from build123d import *

# Parameters (mm, degrees)
SKETCH_1_R          = 2.5
EXTRUDE_1_DEPTH     = 3
SKETCH_2_R          = 1.5
EXTRUDE_2_DEPTH     = 6
CUT_EXTRUDE_1_DEPTH = 2
CHAMFER_1_SIZE      = 0.3
FILLET_1_R          = 0.3


with BuildPart() as part:
    # 草图1 → 凸台-拉伸1 (new body)
    with BuildSketch(Plane.XY):
        Circle(SKETCH_1_R)
    extrude(amount=EXTRUDE_1_DEPTH)

    # 草图2 → 凸台-拉伸2 (add)
    with BuildSketch(Plane(origin=(0, 0, 0), x_dir=(-1, 0, 0), z_dir=(0, 0, -1))):
        Circle(SKETCH_2_R)
    extrude(amount=EXTRUDE_2_DEPTH)

    # 草图3 → 切除-拉伸1 (cut)
    with BuildSketch(Plane.XY.offset(3)):
        Polygon((1.443375673, 0), (0.721687836, 1.25), (-0.721687836, 1.25), (-1.443375673, 0), (-0.721687836, -1.25), (0.721687836, -1.25), align=None)
    extrude(amount=-CUT_EXTRUDE_1_DEPTH, mode=Mode.SUBTRACT)

    # 倒角1
    chamfer_1_edges = [part.edges().sort_by_distance(p)[0] for p in [
        (1.5, 0, -6),
    ]]
    chamfer(chamfer_1_edges, length=CHAMFER_1_SIZE)

    # 圆角1
    fillet_1_edges = [part.edges().sort_by_distance(p)[0] for p in [
        (-2.5, 0, 0),
        (-2.5, 0, 3),
    ]]
    fillet(fillet_1_edges, radius=FILLET_1_R)


solid = part.part
CAD build for the part. Positions are in the model's coordinates, mm. A direction names the side the tool comes from. Give positions to 0.01 mm unless a question says otherwise; leave off trailing zeros. Loops run counter-clockwise (first coordinate to the right, second up) from the corner with the lowest first, then second, coordinate; pieces in that order, holes last. Notation, with made-up numbers: M 6.25,-11.75 L 29.25,-11.75 A23 cw 29.25,27.25 Z; hole C 64.5,-22 d5. An arc over 180 degrees is marked long. Write each question's results on one line, items separated by ' | '.
Q1. Which spindle directions (+Z, -Z, +X, -X, +Y, -Y) get a long thin tool onto all of the face, cutting with end or side? Do faces 1 (the face through (1.088, 0.616, 2.014)), 2 (the face through (-0.03, -1.44, 3)). Say none if no direction does.
Geometry check:
face 1: +Z | face 2: +Z, +X, -X, +Y, -Y
Q2. Band-saw the part on B-B on x = 0. Write the cut outline in (y, z).
Geometry check:
outline: M -2.5,0.3 A0.3 ccw -2.2,0 L -1.5,0 L -1.5,-5.7 L -1.2,-6 L 1.2,-6 L 1.5,-5.7 L 1.5,0 L 2.2,0 A0.3 ccw 2.5,0.3 L 2.5,2.7 A0.3 ccw 2.2,3 L 1.25,3 L 1.25,1 L -1.25,1 L -1.25,3 L -2.2,3 A0.3 ccw -2.5,2.7 Z
Q3. Mould opens along X. For faces 3 (the face through (1.5, 0.07, -2.81)), 4 (the face through (-1.088, -0.616, 2.014)), 5 (the face through (0.9, -1.4, 0)) say: pulls with the +X half, pulls with the -X half, needs draft (parallel to the pull), parting line crosses it, or undercut.
Geometry check:
face 3: parting line crosses it | face 4: undercut | face 5: needs draft
Q4. Probe probe 1 along Z at (x, y) = (0, -1); probe 2 along Z at (x, y) = (1.1, 1.6); probe 3 along Y at (x, z) = (-0.9, -2.25). List the from-to ranges inside material, lowest first.
Geometry check:
probe 1: z = -6 to 1 | probe 2: z = 0 to 3 | probe 3: y = -1.2 to 1.2
Q5. Flat gauge pin, fed straight in: P1, Ø2, axis at x = 1.5, z = -2, coming from the -Y side. Where does the tip first touch, or does it go through?
Geometry check:
P1: stops at y = -1.41
Q6. Band-saw the part on C-C on z = -3. Write the cut outline in (x, y), and give its area (3 significant figures).
Geometry check:
outline: C 0,0 d3 | area: 7.07 mm²
Q7. Band-saw the part on A-A on z = 2.25. Write the cut outline in (x, y).
Geometry check:
outline: C 0,0 d5; hole M -1.44,0 L -0.72,-1.25 L 0.72,-1.25 L 1.44,0 L 0.72,1.25 L -0.72,1.25 Z
